```python
from build123d import *

# Parameters (mm, degrees)
SKETCH2_W                = 5
SKETCH2_H                = 50
BOSS_EXTRUDE1_DEPTH      = 30
BOSS_EXTRUDE1_DEPTH_BACK = 30
SKETCH3_W                = 60
SKETCH3_H                = 12
BOSS_EXTRUDE2_DEPTH      = 42
CUT_EXTRUDE1_REACH       = 49
SKETCH4_R                = 2.25
SKETCH6_R                = 4
CUT_EXTRUDE2_DEPTH       = 2.3
SKETCH7_R                = 2.25
CUT_EXTRUDE3_DEPTH       = 5
SKETCH8_R                = 4
CUT_EXTRUDE4_DEPTH       = 2.3
SKETCH9_R                = 8.15
SKETCH9_R_2              = 4.15
CUT_EXTRUDE5_DEPTH       = 10
CUT_EXTRUDE6_REACH       = 4
SKETCH10_R               = 7.5
SKETCH10_R_2             = 3
CHAMFER1_SIZE            = 14


with BuildPart() as part:
    # Sketch2 → Boss-Extrude1 (new body, two sides)
    with BuildSketch(Plane(origin=(0, 0, 0), x_dir=(0, 0, -1), z_dir=(1, 0, 0))) as boss_extrude1_sk:
        with Locations((13, -32)):
            Rectangle(SKETCH2_W, SKETCH2_H)
    extrude(amount=BOSS_EXTRUDE1_DEPTH)
    extrude(boss_extrude1_sk.sketch, amount=-BOSS_EXTRUDE1_DEPTH_BACK)

    # Sketch3 → Boss-Extrude2 (add)
    with BuildSketch(Plane(origin=(0, 0, -15.5), x_dir=(-1, 0, 0), z_dir=(0, 0, -1))):
        with Locations((0, -51)):
            Rectangle(SKETCH3_W, SKETCH3_H)
    extrude(amount=BOSS_EXTRUDE2_DEPTH)

    # Sketch4 → Cut-Extrude1 (cut, up to next)
    with BuildSketch(Plane.XY.offset(-10.5), mode=Mode.PRIVATE) as cut_extrude1_sk1:
        with Locations((-22.5, -16.75)):
            Circle(SKETCH4_R)
    cut_extrude1_tool1 = extrude(cut_extrude1_sk1.sketch, amount=-CUT_EXTRUDE1_REACH, mode=Mode.PRIVATE) & part.part
    add(cut_extrude1_tool1.solids().sort_by_distance((-22.5, -16.75, -10.5))[0], mode=Mode.SUBTRACT)
    # Sketch4 → Cut-Extrude1 (cut, up to next)
    with BuildSketch(Plane.XY.offset(-10.5), mode=Mode.PRIVATE) as cut_extrude1_sk2:
        with Locations((-7.5, -16.75)):
            Circle(SKETCH4_R)
    cut_extrude1_tool2 = extrude(cut_extrude1_sk2.sketch, amount=-CUT_EXTRUDE1_REACH, mode=Mode.PRIVATE) & part.part
    add(cut_extrude1_tool2.solids().sort_by_distance((-7.5, -16.75, -10.5))[0], mode=Mode.SUBTRACT)
    # Sketch4 → Cut-Extrude1 (cut, up to next)
    with BuildSketch(Plane.XY.offset(-10.5), mode=Mode.PRIVATE) as cut_extrude1_sk3:
        with Locations((7.5, -16.75)):
            Circle(SKETCH4_R)
    cut_extrude1_tool3 = extrude(cut_extrude1_sk3.sketch, amount=-CUT_EXTRUDE1_REACH, mode=Mode.PRIVATE) & part.part
    add(cut_extrude1_tool3.solids().sort_by_distance((7.5, -16.75, -10.5))[0], mode=Mode.SUBTRACT)
    # Sketch4 → Cut-Extrude1 (cut, up to next)
    with BuildSketch(Plane.XY.offset(-10.5), mode=Mode.PRIVATE) as cut_extrude1_sk4:
        with Locations((22.5, -16.75)):
            Circle(SKETCH4_R)
    cut_extrude1_tool4 = extrude(cut_extrude1_sk4.sketch, amount=-CUT_EXTRUDE1_REACH, mode=Mode.PRIVATE) & part.part
    add(cut_extrude1_tool4.solids().sort_by_distance((22.5, -16.75, -10.5))[0], mode=Mode.SUBTRACT)

    # Sketch6 → Cut-Extrude2 (cut)
    with BuildSketch(Plane(origin=(0, 0, -15.5), x_dir=(-1, 0, 0), z_dir=(0, 0, -1))):
        with Locations((-22.5, -16.75)):
            Circle(SKETCH6_R)
        with Locations((-7.5, -16.75)):
            Circle(SKETCH6_R)
        with Locations((7.5, -16.75)):
            Circle(SKETCH6_R)
        with Locations((22.5, -16.75)):
            Circle(SKETCH6_R)
    extrude(amount=-CUT_EXTRUDE2_DEPTH, mode=Mode.SUBTRACT)

    # Sketch7 → Cut-Extrude3 (cut)
    with BuildSketch(Plane.XY.offset(-10.5)):
        with Locations((-24, -52)):
            Circle(SKETCH7_R)
        with Locations((-6, -52)):
            Circle(SKETCH7_R)
        with Locations((-24, -28)):
            Circle(SKETCH7_R)
        with Locations((-6, -28)):
            Circle(SKETCH7_R)
        with Locations((6, -28)):
            Circle(SKETCH7_R)
        with Locations((24, -28)):
            Circle(SKETCH7_R)
        with Locations((6, -52)):
            Circle(SKETCH7_R)
        with Locations((24, -52)):
            Circle(SKETCH7_R)
    extrude(amount=-CUT_EXTRUDE3_DEPTH, mode=Mode.SUBTRACT)

    # Sketch8 → Cut-Extrude4 (cut)
    with BuildSketch(Plane(origin=(0, 0, -15.5), x_dir=(-1, 0, 0), z_dir=(0, 0, -1))):
        with Locations((-24, -28)):
            Circle(SKETCH8_R)
        with Locations((-6, -28)):
            Circle(SKETCH8_R)
        with Locations((6, -28)):
            Circle(SKETCH8_R)
        with Locations((24, -28)):
            Circle(SKETCH8_R)
    extrude(amount=-CUT_EXTRUDE4_DEPTH, mode=Mode.SUBTRACT)

    # Sketch9 → Cut-Extrude5 (cut)
    with BuildSketch(Plane(origin=(0, -45, 0), x_dir=(1, 0, 0), z_dir=(0, 1, 0))):
        with Locations((0, 36.5)):
            Circle(SKETCH9_R)
        with Locations((-20.75, 36.5)):
            Circle(SKETCH9_R_2)
        with Locations((20.75, 36.5)):
            Circle(SKETCH9_R_2)
    extrude(amount=-CUT_EXTRUDE5_DEPTH, mode=Mode.SUBTRACT)

    # Sketch10 → Cut-Extrude6 (cut, up to next)
    with BuildSketch(Plane(origin=(0, -55, 0), x_dir=(1, 0, 0), z_dir=(0, 1, 0)), mode=Mode.PRIVATE) as cut_extrude6_sk1:
        with Locations((0, 36.5)):
            Circle(SKETCH10_R)
    cut_extrude6_tool1 = extrude(cut_extrude6_sk1.sketch, amount=-CUT_EXTRUDE6_REACH, mode=Mode.PRIVATE) & part.part
    add(cut_extrude6_tool1.solids().sort_by_distance((0, -55, -36.5))[0], mode=Mode.SUBTRACT)
    # Sketch10 → Cut-Extrude6 (cut, up to next)
    with BuildSketch(Plane(origin=(0, -55, 0), x_dir=(1, 0, 0), z_dir=(0, 1, 0)), mode=Mode.PRIVATE) as cut_extrude6_sk2:
        with Locations((-20.75, 36.5)):
            Circle(SKETCH10_R_2)
    cut_extrude6_tool2 = extrude(cut_extrude6_sk2.sketch, amount=-CUT_EXTRUDE6_REACH, mode=Mode.PRIVATE) & part.part
    add(cut_extrude6_tool2.solids().sort_by_distance((-20.75, -55, -36.5))[0], mode=Mode.SUBTRACT)
    # Sketch10 → Cut-Extrude6 (cut, up to next)
    with BuildSketch(Plane(origin=(0, -55, 0), x_dir=(1, 0, 0), z_dir=(0, 1, 0)), mode=Mode.PRIVATE) as cut_extrude6_sk3:
        with Locations((20.75, 36.5)):
            Circle(SKETCH10_R_2)
    cut_extrude6_tool3 = extrude(cut_extrude6_sk3.sketch, amount=-CUT_EXTRUDE6_REACH, mode=Mode.PRIVATE) & part.part
    add(cut_extrude6_tool3.solids().sort_by_distance((20.75, -55, -36.5))[0], mode=Mode.SUBTRACT)

    # Chamfer1
    chamfer1_edges = [part.edges().sort_by_distance(p)[0] for p in [
        (30, -51, -57.5),
        (-30, -51, -57.5),
    ]]
    chamfer(chamfer1_edges, length=CHAMFER1_SIZE)


solid = part.part
```
Can you work these out from the model? Positions are in its coordinate system, mm. A direction names the side the tool comes from. Give positions to 0.01 mm unless a question says otherwise; leave off trailing zeros. Order: outer loops, then holes, each group sorted by start corner. A loop starts at its lowest first (then second) coordinate and runs counter-clockwise, first axis right, second up. Notation, with made-up numbers: M 82.25,-22.5 L 91.25,-22.5 A36 ccw 91.25,15.5 Z; hole C -4.5,38.25 d10. An arc over 180 degrees is marked long. Write item = value, one per line. Start each with the question number.
Q1. Suppose I cut it at A-A (y = -52). Write out the boundary of the cut face in (x, z), plus the area to 3 significant figures.
Q2. Suppose I cut it at D-D (z = -25). Write out the boundary of the cut face in (x, y), plus the area to 3 significant figures.
Q3. Will these pins go through, and if not, where does the flat tip stop? pin 1 Ø1 at (x, y) = (2, -39) entering from -Z; pin 2 Ø5 at (x, y) = (6, -28) entering from +Z; pin 3 Ø4 at (x, y) = (-24, -52) entering from +Z; pin 4 Ø6 at (x, y) = (22.5, -16.75) entering from -Z.
Q4. Suppose I cut it at C-C (x = 6). Count the separate pieces of the cut face and the enclosed holes in it, plus the area to 3 significant figures.
Q5. Suppose I cut it at B-B (z = -31.5). Write out the boundary of the cut face in (x, y), plus the area to 3 significant figures.
Q6. We'd pull the mould along Y, two halves only. Please class faces 4 (the cylindrical face through (-6.29, -49.77, -12.96)), 5 (the flat face through (23, -55, -39)), 6 (the cylindrical face through (-1.63, -55.99, -29.18)): pulls with the +Y half, pulls with the -Y half, needs draft (parallel to the pull), parting line crosses it, or undercut.
Q7. For faces 1 (the cylindrical face through (-1.06, -49.93, -44.58)), 2 (the flat face through (-6, -52, -15.5)), 3 (the cylindrical face through (-5.479, -24.034, -14.366)), which set-ups out of +Z, -Z, +X, -X, +Y, -Y let a thin tool reach every point of the face, with its end or its side?
Q8. I need wall thicknesses on probe 1 along Y at (x, z) = (-24, -13.1); probe 2 along Y at (x, z) = (-22.5, -14.95); probe 3 along X at (y, z) = (-48.5, -35). Which ranges of each line are inside material? Lowest first, please. Write a range as [from, to].
Check result:
q1.outline = M -30,-43.5 L -16,-57.5 L 16,-57.5 L 30,-43.5 L 30,-10.5 L 26.25,-10.5 L 26.25,-15.5 L 21.75,-15.5 L 21.75,-10.5 L 8.25,-10.5 L 8.25,-15.5 L 3.75,-15.5 L 3.75,-10.5 L -3.75,-10.5 L -3.75,-15.5 L -8.25,-15.5 L -8.25,-10.5 L -21.75,-10.5 L -21.75,-15.5 L -26.25,-15.5 L -26.25,-10.5 L -30,-10.5 Z; hole C -20.75,-36.5 d8.3; hole C 0,-36.5 d16.3; hole C 20.75,-36.5 d8.3
q1.area = 2,220 mm2
q2.outline = M -30,-57 L 30,-57 L 30,-45 L -30,-45 Z
q2.area = 720 mm2
q3.pin_1 = -15.5
q3.pin_2 = -10.5
q3.pin_3 = -15.5
q3.pin_4 = -13.2
q4.separate_pieces = 4
q4.enclosed_holes = 0
q4.area = 547 mm2
q5.outline = M -30,-57 L -5.59,-57 L -5.59,-55 L -6.44,-55 L -6.44,-45 L -30,-45 Z; M 5.59,-57 L 30,-57 L 30,-45 L 6.44,-45 L 6.44,-55 L 5.59,-55 Z
q5.area = 569 mm2
q6.face_4 = undercut
q6.face_5 = pulls with the +Y half
q6.face_6 = needs draft
q7.face_1 = +Y
q7.face_2 = +Z
q7.face_3 = -Z
q8.probe_1 = [-57, -54.25], [-49.75, -30.25], [-25.75, -18.43], [-15.07, -7]
q8.probe_2 = [-57, -53.68], [-50.32, -31.71], [-24.29, -20.75], [-12.75, -7]
q8.probe_3 = [-30, -24.62], [-16.88, -8.01], [8.01, 16.88], [24.62, 30]
